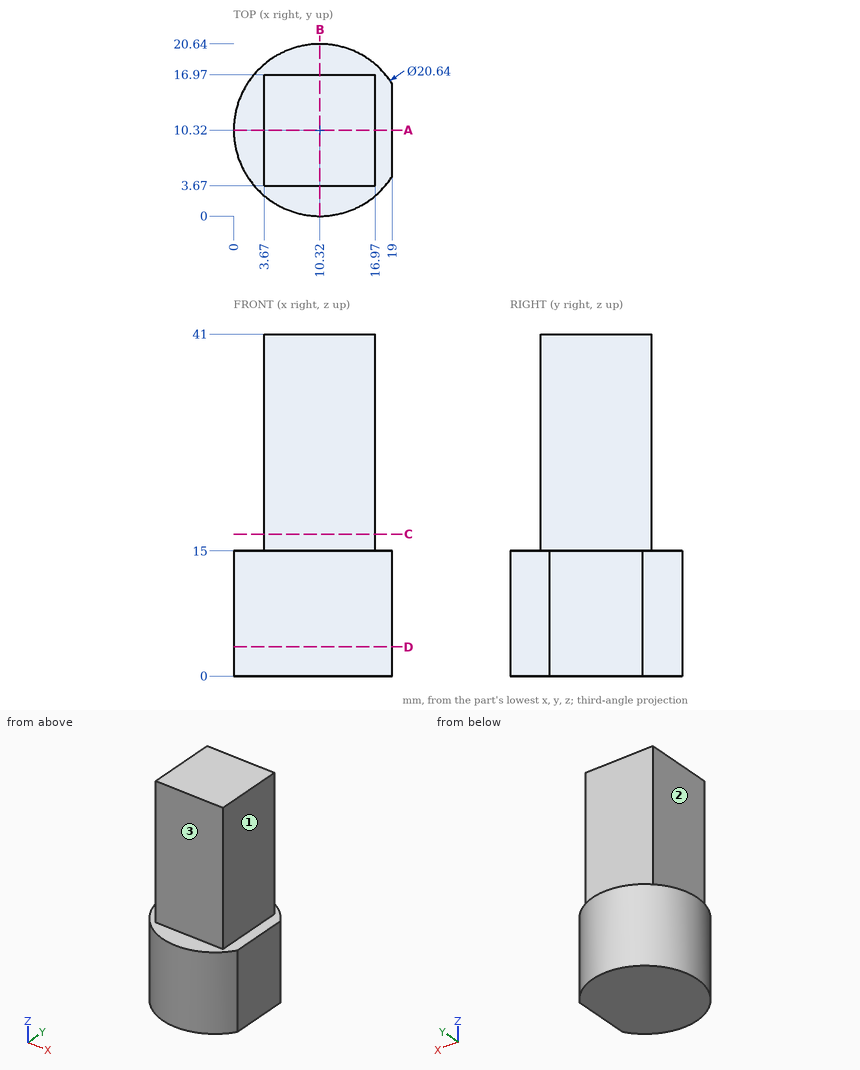
Drawing for the job (mm, zero at the part's lowest x, y, z). A direction names the side the tool comes from. Coordinates: 2 decimals unless noted, no trailing zeros. Order: outer loops, then holes, each group sorted by start corner. A loop starts at its lowest first (then second) coordinate and runs counter-clockwise, first axis right, second up. Notation, with made-up numbers: (-13.5, 18) - (33.5, 18) arc R30 cw to (33.5, 44) - close; hole circle Ø11 at (-11, 89). An arc over 180 degrees is marked (long way). Use a Markdown table: item, result. Add a question column.
(1) Saw through at C-C (z = 17). Give the cut face in (x, y), then the cut area to 3 significant figures.
(2) Drill centre lines: line 1 along Y through (x, z) = (11.5, 20.5); line 2 along Z through (x, y) = (11.5, 17). Where is each one in solid material? Low to high. Write a range as [from, to].
(3) Which spindle directions (+Z, -Z, +X, -X, +Y, -Y) get a long thin tool onto all of the face, cutting with end or side? Do the marked faces 1, 2 and 3. Say none if no direction does.
(4) Saw through at D-D (z = 3.5). Give the cut face in (x, y), then the cut area to 3 significant figures.
(5) Flat gauge pins, fed straight in: pin 1 (2 mm diameter, centred on y = 6, z = 27, fed in from -X); pin 2 (6 mm diameter, centred on y = 12.5, z = 33.5, fed in from +X); pin 3 (10.5 mm diameter, centred on x = 10.5, z = 25, fed in from -Y); pin 4 (3 mm diameter, centred on x = 14, y = 8.5, fed in from -Z). Where does each tip first touch, or does it go through?
(6) Saw through at B-B (x = 10.32). Give the cut face in (y, z), then the cut area to 3 significant figures.
(7) Saw through at A-A (y = 10.32). Give the cut face in (x, z), then the cut area to 3 significant figures.
Solved:
| question | item | result |
|---|---|---|
| 1 | outline | (3.67, 3.67) - (16.97, 3.67) - (16.97, 16.97) - (3.67, 16.97) - close |
| 1 | area | 177 mm² |
| 2 | line 1 | y = [3.67, 16.97] |
| 2 | line 2 | z = [0, 15] |
| 3 | face 1 | +Z, +X, +Y, -Y |
| 3 | face 2 | +Z, -X, +Y, -Y |
| 3 | face 3 | +Z, +X, -X, -Y |
| 4 | outline | (19, 4.74) - (19, 15.9) arc R10.32 ccw (long way) to start |
| 4 | area | 322 mm² |
| 5 | pin 1 | stops at x = 3.67 |
| 5 | pin 2 | stops at x = 16.97 |
| 5 | pin 3 | stops at y = 3.67 |
| 5 | pin 4 | stops at z = 0 |
| 6 | outline | (0, 0) - (20.64, 0) - (20.64, 15) - (16.97, 15) - (16.97, 41) - (3.67, 41) - (3.67, 15) - (0, 15) - close |
| 6 | area | 655 mm² |
| 7 | outline | (0, 0) - (19, 0) - (19, 15) - (16.97, 15) - (16.97, 41) - (3.67, 41) - (3.67, 15) - (0, 15) - close |
| 7 | area | 631 mm² |
